```python
from build123d import *
from OCP.BRepAlgoAPI import BRepAlgoAPI_Cut
from OCP.TopTools import TopTools_ListOfShape

# Parameters (mm, degrees)
SKETCH1_W           = 2200
SKETCH1_H           = 1000
BOSS_EXTRUDE1_DEPTH = 750
SHELL1_T            = -31.75
SCALE1_SCALE        = 0.1
SKETCH36_W          = 3.1749958
SKETCH36_H          = 20.000053956
SKETCH36_W_2        = 3.175
SKETCH36_H_2        = 20
SKETCH36_W_3        = 20
SKETCH36_H_3        = 3.17496467
SKETCH36_H_4        = 3.17503533
CUT_EXTRUDE18_DEPTH = 3.175
SKETCH37_R          = 30
CUT_EXTRUDE19_DEPTH = 3.175
SKETCH38_W          = 3.331279269
SKETCH38_H          = 0.686362951
CUT_EXTRUDE20_DEPTH = 3.175


with BuildPart() as part:
    # Sketch1 → Boss-Extrude1 (new body)
    with BuildSketch(Plane.XY):
        Rectangle(SKETCH1_W, SKETCH1_H)
    extrude(amount=BOSS_EXTRUDE1_DEPTH)

    # Shell1
    shell1_openings = [part.faces().sort_by_distance(p)[0] for p in [
        (0, -500, 375),
        (-1100, 0, 375),
        (0, 500, 375),
        (1100, 0, 375),
        (0, 0, 0),
    ]]
    offset(amount=SHELL1_T, openings=shell1_openings, kind=Kind.INTERSECTION)


with BuildPart() as part_1:
    # Scale1: scaled about (0, 0, 734.125)
    add(part.part.scale(SCALE1_SCALE).moved(Location((0, 0, 660.7125))))


with BuildPart() as cut_extrude18_tool:
    # Sketch36 → Cut-Extrude18 (new body)
    with BuildSketch(Plane.XY.offset(735.7125)):
        with Locations((-108.4125021, 2.6978e-05)):
            Rectangle(SKETCH36_W, SKETCH36_H)
        with Locations((108.4124958, -39.999946044)):
            Rectangle(SKETCH36_W_2, SKETCH36_H_2)
        with Locations((108.4124958, 5.3956e-05)):
            Rectangle(SKETCH36_W_2, SKETCH36_H_2)
        with Locations((108.4124958, 40.000053956)):
            Rectangle(SKETCH36_W_2, SKETCH36_H_2)
        with Locations((-108.4125021, -39.999973022)):
            Rectangle(SKETCH36_W, SKETCH36_H)
        with Locations((-108.4125021, 40.000026978)):
            Rectangle(SKETCH36_W, SKETCH36_H)
        with Locations((39.9999958, 48.412517665)):
            Rectangle(SKETCH36_W_3, SKETCH36_H_3)
        with Locations((79.9999958, 48.412517665)):
            Rectangle(SKETCH36_W_3, SKETCH36_H_3)
        with Locations((-4.2e-06, 48.412517665)):
            Rectangle(SKETCH36_W_3, SKETCH36_H_3)
        with Locations((-40.0000042, 48.412517665)):
            Rectangle(SKETCH36_W_3, SKETCH36_H_3)
        with Locations((-80.0000042, 48.412517665)):
            Rectangle(SKETCH36_W_3, SKETCH36_H_3)
        with Locations((39.9999958, -48.412482335)):
            Rectangle(SKETCH36_W_3, SKETCH36_H_4)
        with Locations((79.9999958, -48.412482335)):
            Rectangle(SKETCH36_W_3, SKETCH36_H_4)
        with Locations((-4.2e-06, -48.412482335)):
            Rectangle(SKETCH36_W_3, SKETCH36_H_4)
        with Locations((-40.0000042, -48.412482335)):
            Rectangle(SKETCH36_W_3, SKETCH36_H_4)
        with Locations((-80.0000042, -48.412482335)):
            Rectangle(SKETCH36_W_3, SKETCH36_H_4)
    extrude(amount=-CUT_EXTRUDE18_DEPTH)


with BuildPart() as part_2:
    add(part_1.part)

    # Cut-Extrude18: cut by cut_extrude18_tool, with a tolerance
    cut_extrude18_stock = TopTools_ListOfShape()
    cut_extrude18_stock.Append(part_2.part.wrapped)
    cut_extrude18_tools = TopTools_ListOfShape()
    cut_extrude18_tools.Append(cut_extrude18_tool.part.wrapped)
    cut_extrude18_cut = BRepAlgoAPI_Cut()
    cut_extrude18_cut.SetArguments(cut_extrude18_stock)
    cut_extrude18_cut.SetTools(cut_extrude18_tools)
    cut_extrude18_cut.SetFuzzyValue(0.00001)
    cut_extrude18_cut.Build()
    add(Compound.cast(cut_extrude18_cut.Shape()).solids(), mode=Mode.REPLACE)

    # Sketch37 → Cut-Extrude19 (cut)
    with BuildSketch(Plane.XY.offset(735.7125)):
        Circle(SKETCH37_R)
    extrude(amount=-CUT_EXTRUDE19_DEPTH, mode=Mode.SUBTRACT)

    # Sketch38 → Cut-Extrude20 (cut)
    with BuildSketch(Plane.XY.offset(735.7125)):
        with Locations((108.490635435, -49.938595097)):
            Rectangle(SKETCH38_W, SKETCH38_H)
    extrude(amount=-CUT_EXTRUDE20_DEPTH, mode=Mode.SUBTRACT)


solid = part_2.part
```
The listing builds one solid part. Answer for the finished solid, in the listing's coordinates (mm). Give positions to 0.01 mm unless a question says otherwise; leave off trailing zeros. Order: outer loops, then holes, each group sorted by start corner. A loop starts at its lowest first (then second) coordinate and runs counter-clockwise, first axis right, second up. Notation, with made-up numbers: M 42,-24.75 L 75,-24.75 A26 ccw 75,14.25 Z; hole C 80,20.5 d6. An arc over 180 degrees is marked long. Put each result on its own line as item: value. Start each with the question number.
Item 1: The part is cut by section D-D, the plane y = -38. Determine the outline of the cut face in (x, z) (1 decimal).
Item 2: The part is cut by section A-A, the plane x = 0. Determine the outline of the cut face in (y, z).
Item 3: The part is cut by section C-C, the plane x = 77.5. Determine the outline of the cut face in (y, z).
Item 4: Find the intervals of material crossed by line 1 along X through (y, z) = (1, 734.5) (3 decimals); line 2 along Y through (x, z) = (0, 734.6); line 3 along Y through (x, z) = (77, 733.55), in increasing order.
Item 5: Flat-ended cylindrical pins translate along their axes: P1, Ø1, axis at y = 48, z = 733.5, coming from the +X side (3 decimals); P2, Ø1, axis at y = -48, z = 734, coming from the -X side (3 decimals). Find the tip coordinate at first contact, or state that the pin passes through.
Item 6: The part is cut by section B-B, the plane y = 0. Determine the outline of the cut face in (x, z) (1 decimal), and give its area (3 significant figures).
Item 7: For a pull along Y with two mould halves and no side action, classify faces 1 (the face through (-26, 23, 735.713)), 2 (the face through (-29.97, 1.32, 734.15)) as +Y half, -Y half, draft (parallel to the pull), parting line (faces both ways), or undercut.
Answer key:
1. outline: M -106.8,732.5 L 106.8,732.5 L 106.8,735.7 L -106.8,735.7 Z
2. outline: M -46.82,732.54 L -30,732.54 L -30,735.71 L -46.82,735.71 Z; M 30,732.54 L 46.83,732.54 L 46.83,735.71 L 30,735.71 Z
3. outline: M -46.82,732.54 L 46.83,732.54 L 46.83,735.71 L -46.82,735.71 Z
4. line 1: x = -106.825 to -29.983, 29.983 to 106.825
4. line 2: y = -46.82 to -30, 30 to 46.83
4. line 3: y = -46.82 to 46.83
5. P1: stops at x = 106.825
5. P2: stops at x = -106.825
6. outline: M -106.8,732.5 L -30,732.5 L -30,735.7 L -106.8,735.7 Z; M 30,732.5 L 106.8,732.5 L 106.8,735.7 L 30,735.7 Z
6. area: 488 mm²
7. face 1: draft
7. face 2: undercut
